Here's the drawing with two shaded views (mm, measured from the low corner). I have some questions. A direction names the side the tool comes from. Round coordinates to 2 decimals unless told otherwise and drop trailing zeros. Write each loop counter-clockwise with the first axis right and the second up, starting at its lowest first coordinate (ties: lowest second). Pieces come first, ordered by that corner, then holes. Notation, with made-up numbers: M -16.75,-17 L 37.25,-17 A18 cw 37.25,-12 Z; hole C 36,74 d1. An arc over 180 degrees is marked long. Write item = value, one per line. Start each with the question number.
(1) On a 3-axis mill with a long thin cutter (end or side, diameter ignored), from which of +Z, -Z, +X, -X, +Y, -Y can I reach the whole of each face in a straight line? I mean the marked faces 5, 6 and 7. Say none if no direction works.
(2) I want a section at A-A (x = 15). List the corners of the cut face in (y, z) for me, and give its area (3 significant figures).
(3) I want a section at B-B (z = 5). List the corners of the cut face in (x, y) for me (1 decimal).
(4) I want a section at D-D (z = 8.75). List the corners of the cut face in (x, y) for me.
(5) If we mould it in two halves opening along Y, with no side actions, what happens to the marked faces 1, 2, 3 and 4? For each: released by +Y, released by -Y, zero draft, split by the parting line, or undercut.
(6) I want a section at C-C (y = 79.5). List the corners of the cut face in (x, z) for me.
(7) Will these pins go through, and if not, where does the flat tip stop? pin 1 Ø3.5 at (x, z) = (5, 5) entering from -Y; pin 2 Ø2 at (x, z) = (11.5, 7.5) entering from -Y; pin 3 Ø11.5 at (x, y) = (15, 49.69) entering from +Z; pin 4 Ø2 at (x, z) = (10.5, 3.5) entering from +Y (1 decimal).
(8) I need wall thicknesses on line 1 along X through (y, z) = (22.5, 5); line 2 along X through (y, z) = (48.5, 5.75); line 3 along X through (y, z) = (46, 5.5) (1 decimal). Which ranges of each line are inside material? Lowest first, please.
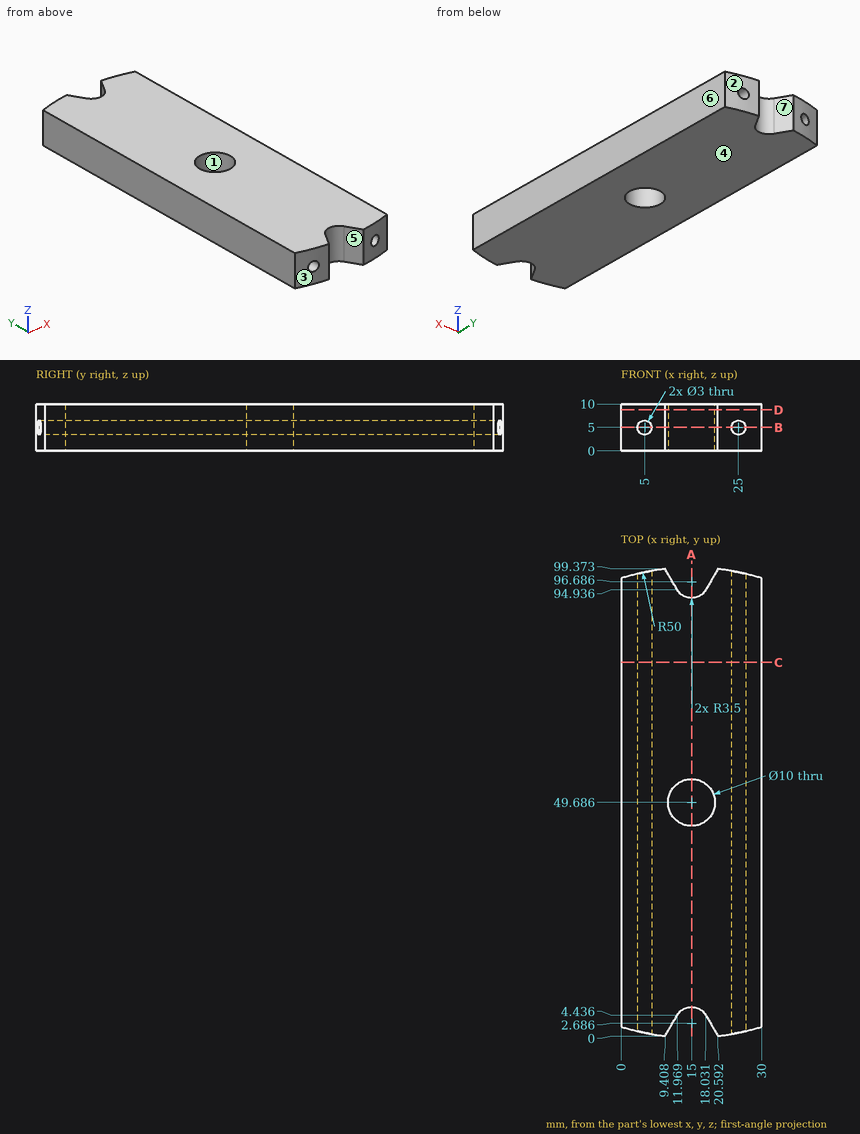
Returned:
q1.face_5 = +Z, -Z, -Y
q1.face_6 = +Z, -Z, +X, +Y, -Y
q1.face_7 = +Z, -Z, +Y
q2.outline = M 6.19,0 L 44.69,0 L 44.69,10 L 6.19,10 Z; M 54.69,0 L 93.19,0 L 93.19,10 L 54.69,10 Z
q2.area = 770 mm²
q3.outline = M 0,2 A50 ccw 3.5,1 L 3.5,98.3 A50 ccw 0,97.4 Z; M 6.5,0.4 A50 ccw 9.4,0 L 12,4.4 A3.5 cw 18,4.4 L 20.6,0 A50 ccw 23.5,0.4 L 23.5,99 A50 ccw 20.6,99.4 L 18,94.9 A3.5 cw 12,94.9 L 9.4,99.4 A50 ccw 6.5,99 Z; M 26.5,1 A50 ccw 30,2 L 30,97.4 A50 ccw 26.5,98.3 Z; hole C 15,49.7 d10
q4.outline = M 0,1.99 A50 ccw 9.41,0 L 11.97,4.44 A3.5 cw 18.03,4.44 L 20.59,0 A50 ccw 30,1.99 L 30,97.38 A50 ccw 20.59,99.37 L 18.03,94.94 A3.5 cw 11.97,94.94 L 9.41,99.37 A50 ccw 0,97.38 Z; hole C 15,49.69 d10
q5.face_1 = undercut
q5.face_2 = released by +Y
q5.face_3 = released by -Y
q5.face_4 = zero draft
q6.outline = M 0,0 L 30,0 L 30,10 L 0,10 Z; hole C 5,5 d3; hole C 25,5 d3
q7.pin_1 = 0.37
q7.pin_2 = 1.89
q7.pin_3 = 10
q7.pin_4 = 99.2
q8.line_1 = 0 to 3.5, 6.5 to 23.5, 26.5 to 30
q8.line_2 = 0 to 3.7, 6.3 to 10.14, 19.86 to 23.7, 26.3 to 30
q8.line_3 = 0 to 3.6, 6.4 to 11.6, 18.4 to 23.6, 26.4 to 30
